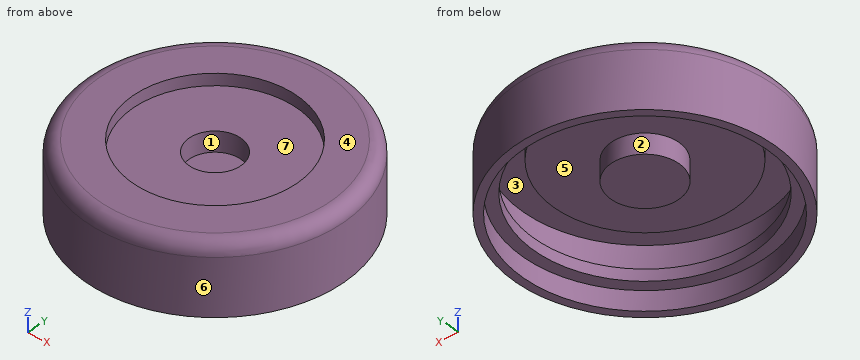
from build123d import *


with BuildPart() as f1:
    # F0 (on Front) → F1 (revolve)
    with BuildSketch(Plane.XZ):
        with BuildLine():
            Line((-49.135093, 21.603222), (-49.135093, 0))
            Line((-49.135093, 0), (-46.135093, 0))
            Line((-46.135093, 0), (-46.135093, 7.41767))
            Line((-46.135093, 7.41767), (-41.773196, 7.41767))
            Line((-41.773196, 7.41767), (-41.773196, 11.801611))
            Line((-41.773196, 11.801611), (-46.135093, 11.801611))
            Line((-46.135093, 11.801611), (-46.135093, 23.603222))
            Line((-46.135093, 23.603222), (-34.280277, 23.603222))
            Line((-34.280277, 23.603222), (-34.280277, 19.141468))
            Line((-34.280277, 19.141468), (-12.863847, 19.141468))
            Line((-12.863847, 19.141468), (-12.863847, 11.556481))
            Line((-12.863847, 11.556481), (0, 11.556481))
            Line((0, 11.556481), (0, 14.556481))
            Line((0, 14.556481), (-9.863847, 14.556481))
            Line((-9.863847, 14.556481), (-9.863847, 22.141468))
            Line((-9.863847, 22.141468), (-31.280277, 22.141468))
            Line((-31.280277, 22.141468), (-31.280277, 26.603222))
            Line((-31.280277, 26.603222), (-44.135093, 26.603222))
            ThreePointArc((-44.135093, 26.603222), (-47.670627, 25.138756), (-49.135093, 21.603222))
        make_face()
    revolve(axis=Axis((0, 0, 13.056481), (0, 0, -1)))


solid = f1.part
Here's how the part is built. I have some questions about the finished solid (model axes, mm). Face numbers are marked on the shaded views. A direction names the side the tool comes from. Give positions to 0.01 mm unless a question says otherwise; leave off trailing zeros. Write each loop counter-clockwise with the first axis right and the second up, starting at its lowest first coordinate (ties: lowest second). Pieces come first, ordered by that corner, then holes. Notation, with made-up numbers: (63.5, 70.5) -> (97.5, 70.5) arc R12 cw to (97.5, 74.5) -> close; hole circle Ø8 at (38.25, 59.25). An arc over 180 degrees is marked (long way). Use one line per item in the form item = value. Start each with the question number.
1. Imagine slicing it at D-D on z = 4.25. List the corners of the cut face in (x, y) for me, plus the area to 3 significant figures.
2. On a 3-axis mill with a long thin cutter (end or side, diameter ignored), from which of +Z, -Z, +X, -X, +Y, -Y can I reach the whole of each face in a straight line? I mean the marked faces 1, 2 and 3. Say none if no direction works.
3. Will these pins go through, and if not, where does the flat tip stop? pin 1 Ø18 at (x, y) = (0, 0) entering from +Z; pin 2 Ø10 at (x, z) = (28.5, 20.5) entering from +Y; pin 3 Ø12 at (x, y) = (-2.5, 32) entering from -Z.
4. If I drill on L1, parallel to Y at x = 0, z = 16.5; L2, parallel to Y at x = 0, z = 5.5; L3, parallel to Y at x = -3.5, z = 22, over which ranges is the centre line in solid material (lowest first)?
5. Imagine slicing it at B-B on z = 17.75. List the corners of the cut face in (x, y) for me, plus the area to 3 significant figures.
6. Thinking about a two-plate mould opening in Y: for the marked faces 4, 5, 6 and 7, which applies, +Y half, -Y half, draft (parallel to the pull), parting line (faces both ways), or undercut?
Entries:
q1.outline = circle Ø98.27 at (0, 0); hole circle Ø92.27 at (0, 0)
q1.area = 898 mm²
q2.face_1 = +Z
q2.face_2 = -Z
q2.face_3 = none
q3.pin_1 = 14.56
q3.pin_2 = 43.15
q3.pin_3 = 19.14
q4.L1 = -49.14 to -46.14, -12.86 to -9.86, 9.86 to 12.86, 46.14 to 49.14
q4.L2 = -49.14 to -46.14, 46.14 to 49.14
q4.L3 = -48.99 to -46, -34.1 to -9.22, 9.22 to 34.1, 46 to 48.99
q5.outline = circle Ø98.27 at (0, 0); circle Ø25.73 at (0, 0); hole circle Ø92.27 at (0, 0); hole circle Ø19.73 at (0, 0)
q5.area = 1,110 mm²
q6.face_4 = draft
q6.face_5 = undercut
q6.face_6 = parting line
q6.face_7 = undercut
